```python
from build123d import *

# Parameters (mm, degrees)
SKETCH1_R           = 42.926
SKETCH1_R_2         = 39.751
BOSS_EXTRUDE1_DEPTH = 7.62
SKETCH2_R           = 1.7526
CUT_EXTRUDE1_DEPTH  = 95.7
CIRPATTERN1_COUNT   = 8
SKETCH6_R           = 1.7526
CUT_EXTRUDE2_DEPTH  = 119.35
BOSS_EXTRUDE2_START = -7.62
SKETCH8_W           = 6.519417161
SKETCH8_H           = 7.62
BOSS_EXTRUDE2_DEPTH = 12
SKETCH10_R          = 1.7526
CUT_EXTRUDE3_DEPTH  = 9
CIRPATTERN2_COUNT   = 2


with BuildPart() as part:
    # Sketch1 → Boss-Extrude1 (new body)
    # profile 1 of 3: a face of its own
    with BuildSketch(Plane(origin=(0, 0, 0), x_dir=(1, 0, 0), z_dir=(0, 1, 0))):
        with BuildLine():
            Line((-167.759899912, -119.886046801), (-167.759899912, -127.506046801))
            Line((-167.759899912, -127.506046801), (-161.24048275, -127.506046801))
            ThreePointArc((-161.24048275, -127.506046801), (-161.409899912, -123.696046801), (-161.24048275, -119.886046801))
            Line((-161.24048275, -119.886046801), (-167.759899912, -119.886046801))
        make_face()
    # profile 2 of 3: a face of its own
    with BuildSketch(Plane(origin=(0, 0, 0), x_dir=(1, 0, 0), z_dir=(0, 1, 0))):
        with Locations((-118.483899912, -123.696046801)):
            Circle(SKETCH1_R)
        with Locations(Location((-118.483899912, -123.696046801, 0), (0, 0, 90))):
            Circle(SKETCH1_R_2, mode=Mode.SUBTRACT)
    # profile 3 of 3: a face of its own
    with BuildSketch(Plane(origin=(0, 0, 0), x_dir=(1, 0, 0), z_dir=(0, 1, 0))):
        with BuildLine():
            ThreePointArc((-75.557899912, -123.696046801), (-75.600275118, -125.602929216), (-75.727317073, -127.506046801))
            Line((-75.727317073, -127.506046801), (-69.207899912, -127.506046801))
            Line((-69.207899912, -127.506046801), (-69.207899912, -119.886046801))
            Line((-69.207899912, -119.886046801), (-75.727317073, -119.886046801))
            ThreePointArc((-75.727317073, -119.886046801), (-75.600275118, -121.789164387), (-75.557899912, -123.696046801))
        make_face()
    extrude(amount=BOSS_EXTRUDE1_DEPTH)

    # Sketch2 → Cut-Extrude1 (cut)
    with BuildSketch(Plane.XY):
        with Locations(Location((-118.483899912, 3.81, 0), (0, 0, 180))):
            Circle(SKETCH2_R)
    cut_extrude1 = extrude(amount=CUT_EXTRUDE1_DEPTH, mode=Mode.SUBTRACT)

    # CirPattern1: Cut-Extrude1 ×8 about axis, 2 skipped
    cirpattern1_axis = Axis((-118.483899912, 7.62, 123.696046801), (0, 1, 0))
    add([cut_extrude1.rotate(cirpattern1_axis, i * 360 / CIRPATTERN1_COUNT) for i in range(1, CIRPATTERN1_COUNT) if i not in (2, 6)], mode=Mode.SUBTRACT)

    # Sketch6 → Cut-Extrude2 (cut)
    with BuildSketch(Plane.ZY.offset(167.759899912)):
        with Locations((123.696046801, 3.877276016)):
            Circle(SKETCH6_R)
    extrude(amount=-CUT_EXTRUDE2_DEPTH, mode=Mode.SUBTRACT)

    # Sketch8 → Boss-Extrude2 (add)
    with BuildSketch(Plane(origin=(0, 7.62, 0), x_dir=(1, 0, 0), z_dir=(0, 1, 0)).offset(BOSS_EXTRUDE2_START)):
        with Locations((-72.467608493, -123.696046801)):
            Rectangle(SKETCH8_W, SKETCH8_H)
    boss_extrude2 = extrude(amount=-BOSS_EXTRUDE2_DEPTH)

    # Sketch10 → Cut-Extrude3 (cut)
    with BuildSketch(Plane(origin=(-69.207899912, 0, 0), x_dir=(0, 0, -1), z_dir=(1, 0, 0))):
        with Locations((-123.683858545, -8.849612584)):
            Circle(SKETCH10_R)
    cut_extrude3 = extrude(amount=-CUT_EXTRUDE3_DEPTH, mode=Mode.SUBTRACT)

    # CirPattern2: Boss-Extrude2, Cut-Extrude3 ×2 about axis
    cirpattern2_axis = Axis((-118.483899912, 7.62, 123.696046801), (0, 1, 0))
    add([boss_extrude2.rotate(cirpattern2_axis, i * 360 / CIRPATTERN2_COUNT) for i in range(1, CIRPATTERN2_COUNT)])
    add([cut_extrude3.rotate(cirpattern2_axis, i * 360 / CIRPATTERN2_COUNT) for i in range(1, CIRPATTERN2_COUNT)], mode=Mode.SUBTRACT)


solid = part.part
```
Design review of the part built by this model. Coordinates are the model's own, in mm. A direction names the side the tool comes from. Give positions to 0.01 mm unless a question says otherwise; leave off trailing zeros. Write each loop counter-clockwise with the first axis right and the second up, starting at its lowest first coordinate (ties: lowest second). Pieces come first, ordered by that corner, then holes. Notation, with made-up numbers: (78, 78.5) - (109, 78.5) arc R8 ccw to (109, 89.5) - close; hole circle Ø9 at (26, 85). An arc over 180 degrees is marked (long way). Return JSON: item names as keys, results as strings. Group by question number.
(1) We need section C-C, the plane x = -77.5. Give the boundary of the cut face in (y, z).
(2) Insertion check: pin 1 (4.5 mm diameter, centred on x = -118.48, y = 3.81, fed in from -Z); pin 2 (2 mm diameter, centred on x = -163.5, y = 0, fed in from +Z); pin 3 (2 mm diameter, centred on y = 3.5, z = 145.5, fed in from -X); pin 4 (2 mm diameter, centred on y = 3.88, z = 123.7, fed in from -X). Each pin has a flat end and moves straight along its axis. Give the tip position at first contact, or say it passes through.
(3) Mouldability with a two-part tool opening along X and no side actions: class faces 1 (the cylindrical face through (-117.59, 2.06, 80.78)), 2 (the cylindrical face through (-89.823, 5.365, 93.891)), 3 (the flat face through (-73, -2, 127.506)) as +X half, -X half, draft (parallel to the pull), parting line (faces both ways), or undercut.
(4) To check wall thickness, follow probe 1 along X at (y, z) = (-10.5, 121); probe 2 along Z at (x, y) = (-104.5, 2.75); probe 3 along X at (y, z) = (3.25, 92). State the ranges of each line that lie inside material, in increasing order.
(5) We need section A-A, the plane y = -2. Give the boundary of the cut face in (x, z), then the cut area to 3 significant figures.
(6) We need section B-B, the plane z = 110. Give the boundary of the cut face in (x, y).
(7) Machinability: for faces 4 (the cylindrical face through (-103.259, 3.757, 86.976)), 5 (the flat face through (-75.727, -6, 124)), 6 (the flat face through (-73, -2, 119.886)), which of the approach directions +Z, -Z, +X, -X, +Y, -Y give a long, thin tool a straight path to every point of the face, cutting with its end or side? Answer none if there is none.
Reported:
{
 "1": {"outline": "(0, 110.93) - (7.62, 110.93) - (7.62, 136.46) - (0, 136.46) - close; hole circle Ø3.51 at (3.88, 123.7)"},
 "2": {"pin 1": "stops at z = 80.77", "pin 2": "stops at z = 127.51", "pin 3": "stops at x = -156.03", "pin 4": "passes through"},
 "3": {"face 1": "parting line", "face 2": "undercut", "face 3": "draft"},
 "4": {"probe 1": "x = -167.76 to -161.24, -75.73 to -69.21", "probe 2": "z = 83.11 to 86.49, 160.91 to 164.28", "probe 3": "x = -147.43 to -142.47, -94.49 to -89.54"},
 "5": {"outline": "(-167.76, 119.89) - (-161.24, 119.89) - (-161.24, 127.51) - (-167.76, 127.51) - close; (-75.73, 119.89) - (-69.21, 119.89) - (-69.21, 127.51) - (-75.73, 127.51) - close", "area": "99.4 mm2"},
 "6": {"outline": "(-159.17, 0) - (-155.8, 0) - (-155.8, 7.62) - (-159.17, 7.62) - close; (-81.17, 0) - (-77.8, 0) - (-77.8, 7.62) - (-81.17, 7.62) - close"},
 "7": {"face 4": "+Y, -Y", "face 5": "+Z, -Z, -Y", "face 6": "-Z, +X, +Y, -Y"}
}
